Work out the finished part from the listing and answer in its coordinate system (mm). A direction names the side the tool comes from. Round coordinates to 2 decimals unless told otherwise and drop trailing zeros. Loops run counter-clockwise (first coordinate to the right, second up) from the corner with the lowest first, then second, coordinate; pieces in that order, holes last. Notation, with made-up numbers: (31.25, 68) -> (46.25, 68) arc R19 cw to (46.25, 103) -> close; hole circle Ø1 at (42, 22.25). An arc over 180 degrees is marked (long way). Use one line per item in the form item = value.
```python
from build123d import *

# Parameters (mm, degrees)
BOSS_EXTRUDE1_DEPTH = 30
SKETCH2_R           = 2.5
CUT_EXTRUDE1_DEPTH  = 30


with BuildPart() as part:
    # Sketch1 → Boss-Extrude1 (new body)
    with BuildSketch(Plane.XY):
        with BuildLine():
            Line((89.932901242, 3.47466175), (99.749159056, 3.47466175))
            Line((99.749159056, 3.47466175), (99.749159056, -6.52533825))
            Line((99.749159056, -6.52533825), (84.749159056, -6.52533825))
            ThreePointArc((84.749159056, -6.52533825), (0, 85), (-84.749159056, -6.52533825))
            Line((-84.749159056, -6.52533825), (-99.749159056, -6.52533825))
            Line((-99.749159056, -6.52533825), (-99.749159056, 3.47466175))
            Line((-99.749159056, 3.47466175), (-89.932901242, 3.47466175))
            ThreePointArc((-89.932901242, 3.47466175), (0, 90), (89.932901242, 3.47466175))
        make_face()
    extrude(amount=BOSS_EXTRUDE1_DEPTH)

    # Sketch2 → Cut-Extrude1 (cut)
    with BuildSketch(Plane(origin=(0, 3.47466175, 0), x_dir=(1, 0, 0), z_dir=(0, 1, 0))):
        with Locations(Location((-94.841030149, -10, 0), (0, 0, 180))):
            Circle(SKETCH2_R)
        with Locations(Location((-94.841030149, -20, 0), (0, 0, 180))):
            Circle(SKETCH2_R)
        with Locations(Location((94.841030149, -20, 0), (0, 0, 180))):
            Circle(SKETCH2_R)
        with Locations(Location((94.841030149, -10, 0), (0, 0, 180))):
            Circle(SKETCH2_R)
    extrude(amount=-CUT_EXTRUDE1_DEPTH, mode=Mode.SUBTRACT)


solid = part.part
```
(1) For a pull along Z with two mould halves and no side action, classify faces 3 (the cylindrical face through (-97.226, -1.455, 20.751)), 4 (the cylindrical face through (96.825, -1.455, 8.479)), 5 (the flat face through (95, 3.475, 15)), 6 (the flat face through (-7, 85, 0)) as +Z half, -Z half, draft (parallel to the pull), parting line (faces both ways), or undercut.
Completed:
face_3 = undercut
face_4 = undercut
face_5 = draft
face_6 = -Z half
(2) Find section C-C, the plane y = 14. Write down the section's boundary in (x, z).
Completed:
outline = (-88.9, 0) -> (-83.84, 0) -> (-83.84, 30) -> (-88.9, 30) -> close; (83.84, 0) -> (88.9, 0) -> (88.9, 30) -> (83.84, 30) -> close
(3) Given P1, Ø2, axis at x = 3, z = 4, coming from the +Y side; P2, Ø10, axis at x = 45, z = 23.5, coming from the +Y side; P3, Ø6, axis at x = 27, z = 17, coming from the -Y side; P4, Ø8, axis at x = 94.84, z = 20, coming from the -Y side, each flat-ended and moving along its own axis, determine where each tip first touches the part or whether it passes through.
Completed:
P1 = 89.98
P2 = 80.62
P3 = 79.53
P4 = -6.53
(4) Consider L1, parallel to X at y = -1, z = 13.5; L2, parallel to X at y = 32.5, z = 20; L3, parallel to Y at x = -43, z = 4.25. Determine where each line is inside the solid, lowest interval first.
Completed:
L1 = -99.75 to -84.99, 84.99 to 99.75
L2 = -83.93 to -78.54, 78.54 to 83.93
L3 = 73.32 to 79.06
(5) For faces 1 (the cylindrical face through (-1.93, 89.98, 14.79)), 2 (the flat face through (-95, 3.475, 15)), determine the directions among +Z, -Z, +X, -X, +Y, -Y from which every point of the face is accessible in a straight line to the end or side of a thin tool.
Completed:
face_1 = +Z, -Z, +Y
face_2 = +Z, -Z, -X, +Y
(6) Find section A-A, the plane y = 0. Write down the section's boundary in (x, z).
Completed:
outline = (-99.75, 0) -> (-85, 0) -> (-85, 30) -> (-99.75, 30) -> close; (85, 0) -> (99.75, 0) -> (99.75, 30) -> (85, 30) -> close; hole circle Ø5 at (-94.84, 10); hole circle Ø5 at (-94.84, 20); hole circle Ø5 at (94.84, 10); hole circle Ø5 at (94.84, 20)
(7) Find section D-D, the plane x = 0. Write down the section's boundary in (y, z), then the cut area to 3 significant figures.
Completed:
outline = (85, 0) -> (90, 0) -> (90, 30) -> (85, 30) -> close
area = 150 mm2
